Work out the finished part from the listing and answer in its coordinate system (mm). Face numbers are marked on the shaded views. A direction names the side the tool comes from. Coordinates: 2 decimals unless noted, no trailing zeros. Order: outer loops, then holes, each group sorted by start corner. A loop starts at its lowest first (then second) coordinate and runs counter-clockwise, first axis right, second up.
1. The part is cut by section B-B, the plane y = -435.5. Give the vertices of the cut face in (x, z).
2. Determine the mould class of the marked faces 1, 2, 3 and 4 for opening direction X: +X half, -X half, draft (parallel to the pull), parting line (faces both ways), or undercut.
3. Find the intervals of material crossed by probe 1 along X at (y, z) = (-246.5, -547); probe 2 along X at (y, z) = (-363.5, -200), in increasing order.
4. The part is cut by section C-C, the plane x = -69.5. Give the vertices of the cut face in (y, z), then the cut area to 3 significant figures.
5. The part is cut by section A-A, the plane z = -462.5. Give the vertices of the cut face in (x, y).
6. The part is cut by section D-D, the plane z = 98.5. Give the vertices of the cut face in (x, y), then the cut area to 3 significant figures.
7. Flat-ended cylindrical pins translate along their axes: pin 1 Ø1 at (y, z) = (29.5, -6.5) entering from +X; pin 2 Ø5 at (x, z) = (245, -296) entering from +Y; pin 3 Ø3 at (y, z) = (142.5, -21) entering from -X. Find the tip coordinate at first contact, or state that the pin passes through.
8. A tool of negligible diameter and unlimited length cuts with its end or side. For the marked faces 5, 6 and 7, from which of +Z, -Z, +X, -X, +Y, -Y can it reach the whole face along a straight path? Write none if from no direction.
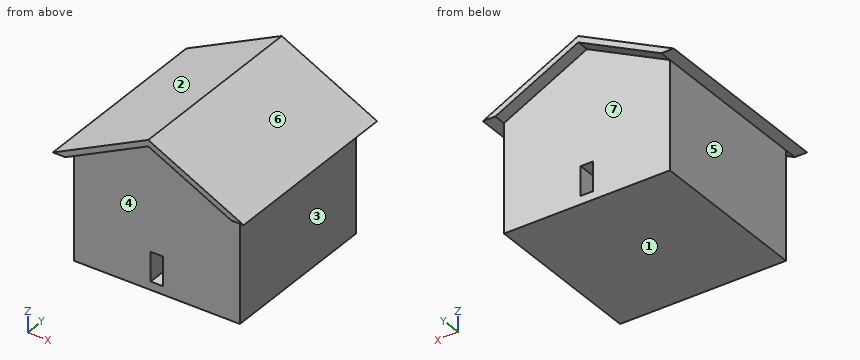
```python
from build123d import *

# Parameters (mm, degrees)
F1_DEPTH = 584.2
F0_W     = 469.9
F0_H     = 50.8
F2_DEPTH = 508


with BuildPart() as f1:
    # F0 (on Front) → F1 (new body, symmetric)
    with BuildSketch(Plane.XZ):
        Polygon((-584.2, 0), (-508, 0), (0, 254), (0, 292.1), align=None)
        Polygon((0, 254), (508, 0), (584.2, 0), (0, 292.1), align=None)
    extrude(amount=F1_DEPTH, both=True)

    # F0 (on Front) → F2 (join, symmetric)
    with BuildSketch(Plane.XZ):
        Polygon((508, 0), (0, 0), (-508, 0), (-508, -609.6), (-38.1, -609.6), (-38.1, -431.8), (38.1, -431.8), (38.1, -609.6), (508, -609.6), align=None)
        Polygon((0, 254), (0, 0), (508, 0), align=None)
        Polygon((-508, 0), (0, 0), (0, 254), align=None)
        Polygon((-584.2, 0), (-508, 0), (0, 254), (0, 292.1), align=None)
        Polygon((0, 254), (508, 0), (584.2, 0), (0, 292.1), align=None)
        with Locations((-273.05, -635)):
            Rectangle(F0_W, F0_H)
        with Locations((273.05, -635)):
            Rectangle(F0_W, F0_H)
        Polygon((0, -609.6), (-38.1, -609.6), (-38.1, -660.4), (38.1, -660.4), (38.1, -609.6), align=None)
    extrude(amount=F2_DEPTH, both=True)


solid = f1.part
```
Geometry says:
1. outline: (-584.2, 0) - (-508, 0) - (-508, -660.4) - (508, -660.4) - (508, 0) - (584.2, 0) - (0, 292.1) - close; hole (-38.1, -609.6) - (38.1, -609.6) - (38.1, -431.8) - (-38.1, -431.8) - close
2. face 1: draft
2. face 2: -X half
2. face 3: +X half
2. face 4: undercut
3. probe 1: x = -508 to -38.1, 38.1 to 508
3. probe 2: x = -508 to 508
4. outline: (-584.2, 219.25) - (-508, 219.25) - (-508, -660.4) - (508, -660.4) - (508, 219.25) - (584.2, 219.25) - (584.2, 257.35) - (-584.2, 257.35) - close
4. area: 938,000 mm2
5. outline: (-508, -508) - (-38.1, -508) - (-38.1, 508) - (-508, 508) - close; (38.1, -508) - (508, -508) - (508, 508) - (38.1, 508) - close
6. outline: (-387.2, -584.2) - (-311, -584.2) - (-311, -508) - (311, -508) - (311, -584.2) - (387.2, -584.2) - (387.2, 584.2) - (311, 584.2) - (311, 508) - (-311, 508) - (-311, 584.2) - (-387.2, 584.2) - close
6. area: 810,000 mm2
7. pin 1: stops at x = 508
7. pin 2: stops at y = 508
7. pin 3: stops at x = -508
8. face 5: -Z, -X, +Y, -Y
8. face 6: +Z, +X, +Y, -Y
8. face 7: -Z, +Y
